Design review of the part shown in the three views and the two pictorial views. Dimensions are in mm from the part's minimum x, y and z. Round coordinates to 2 decimals unless told otherwise and drop trailing zeros. Write each loop counter-clockwise with the first axis right and the second up, starting at its lowest first coordinate (ties: lowest second). Pieces come first, ordered by that corner, then holes. Notation, with made-up numbers: (58.25, 54.25) - (84.25, 54.25) arc R16 ccw to (84.25, 74.25) - close; hole circle Ø6 at (-3, 4). An arc over 180 degrees is marked (long way). Use one line per item in the form item = value.
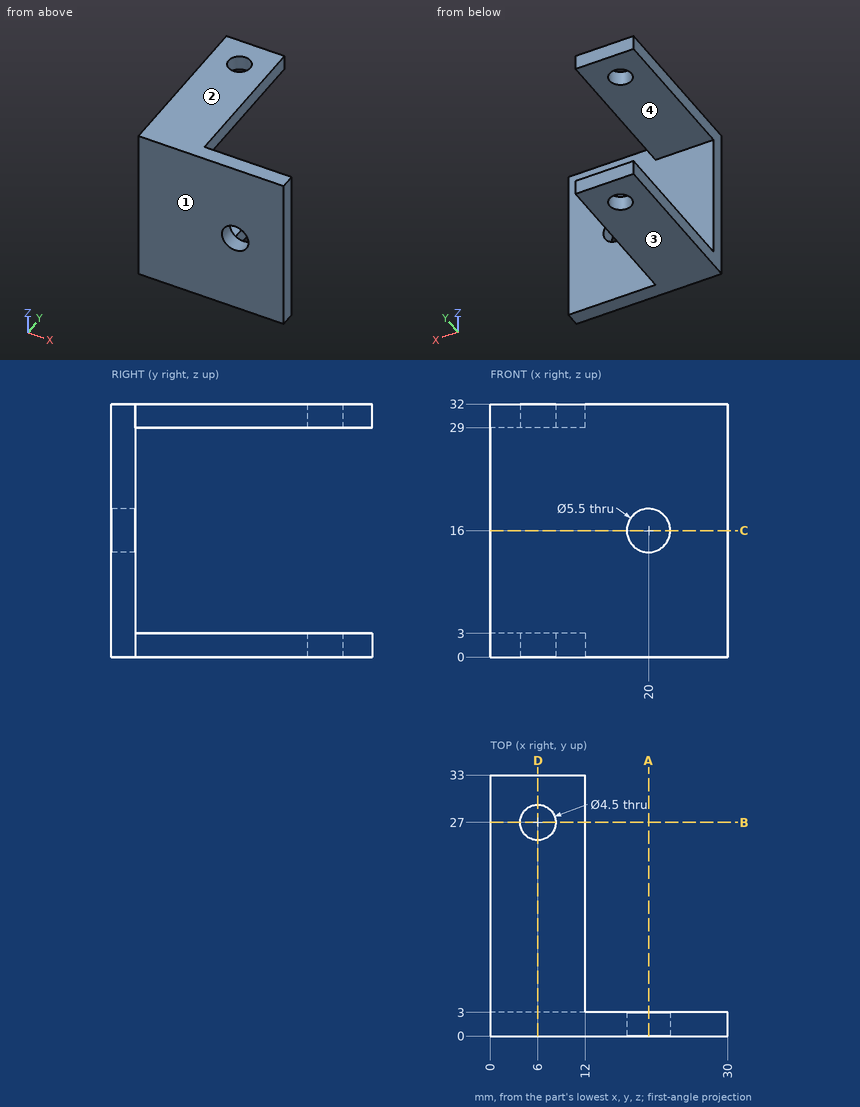
(1) Add section C-C on z = 16. Write out the cut boundary in (x, y).
Geometry results:
outline = (0, 0) - (17.25, 0) - (17.25, 3) - (0, 3) - close; (22.75, 0) - (30, 0) - (30, 3) - (22.75, 3) - close
(2) Insertion check: P1, Ø9, axis at x = 20, z = 16, coming from the +Y side; P2, Ø1.5, axis at y = 12.5, z = 30.5, coming from the +X side; P3, Ø13, axis at x = 7, y = 21, coming from the -Z side. Each pin has a flat end and moves straight along its axis. Give the tip position at first contact, or say it passes through.
Geometry results:
P1 = 3
P2 = 12
P3 = 0
(3) Add section A-A on x = 20. Write out the cut boundary in (y, z).
Geometry results:
outline = (0, 0) - (3, 0) - (3, 13.25) - (0, 13.25) - close; (0, 18.75) - (3, 18.75) - (3, 32) - (0, 32) - close
(4) The part is to be moulded in two halves that separate along Z. For the marked faces 1, 2, 3 and 4, say which applies: +Z half, -Z half, draft (parallel to the pull), parting line (faces both ways), or undercut.
Geometry results:
face_1 = draft
face_2 = +Z half
face_3 = -Z half
face_4 = undercut
(5) Add section D-D on x = 6. Write out the cut boundary in (y, z), then the cut area to 3 significant figures.
Geometry results:
outline = (0, 0) - (24.75, 0) - (24.75, 3) - (3, 3) - (3, 29) - (24.75, 29) - (24.75, 32) - (0, 32) - close; (29.25, 0) - (33, 0) - (33, 3) - (29.25, 3) - close; (29.25, 29) - (33, 29) - (33, 32) - (29.25, 32) - close
area = 249 mm2
(6) To check wall thickness, follow L1, parallel to X at y = 1.9, z = 16; L2, parallel to Y at x = 6, z = 2; L3, parallel to Z at x = 11.25, y = 29. State the ranges of each line that lie inside material, in increasing order.
Geometry results:
L1 = 0 to 17.25, 22.75 to 30
L2 = 0 to 24.75, 29.25 to 33
L3 = 0 to 3, 29 to 32
(7) Add section B-B on y = 27. Write out the cut boundary in (x, z).
Geometry results:
outline = (0, 0) - (3.75, 0) - (3.75, 3) - (0, 3) - close; (0, 29) - (3.75, 29) - (3.75, 32) - (0, 32) - close; (8.25, 0) - (12, 0) - (12, 3) - (8.25, 3) - close; (8.25, 29) - (12, 29) - (12, 32) - (8.25, 32) - close
